Can you work these out from the model? Positions are in its coordinate system, mm. Face numbers are marked on the shaded views. A direction names the side the tool comes from. Give positions to 0.01 mm unless a question says otherwise; leave off trailing zeros. Order: outer loops, then holes, each group sorted by start corner. A loop starts at its lowest first (then second) coordinate and runs counter-clockwise, first axis right, second up. Notation, with made-up numbers: M 31,43 L 69,43 A31 cw 69,78 Z; hole C 64,37.25 d11. An arc over 180 degrees is marked long. Write each question's results on one line, items separated by ' | '.
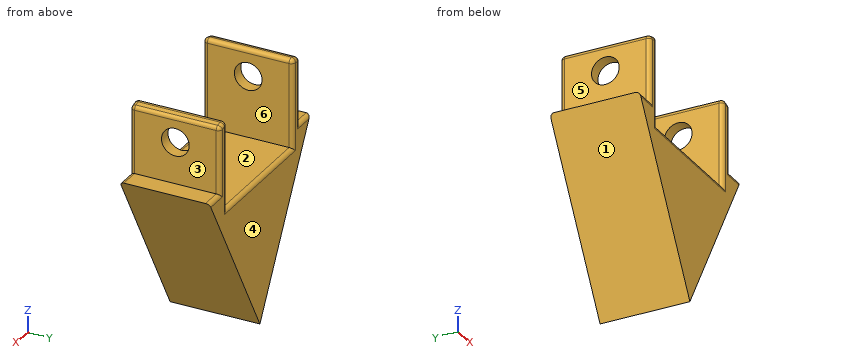
from build123d import *

# Parameters (mm, degrees)
BOSS_EXTRUDE1_DEPTH = 28
CUT_EXTRUDE1_DEPTH  = 90.677477663
SKETCH5_R           = 6.35
CUT_EXTRUDE2_DEPTH  = 4.572
SKETCH8_R           = 6.35
SKETCH8_R_2         = 4.318
BOSS_EXTRUDE4_DEPTH = 6.858
CUT_EXTRUDE6_START  = -2.54
SKETCH13_W          = 36.221601717
SKETCH13_H          = 27.797973411
CUT_EXTRUDE6_DEPTH  = 91.021953984
FILLET3_R           = 1.27


with BuildPart() as part:
    # Sketch2 → Boss-Extrude1 (new body)
    with BuildSketch(Plane(origin=(0, 0, 0), x_dir=(1, 0, 0), z_dir=(0, 1, 0))):
        with BuildLine():
            Line((-38.1, -65.991135768), (0, 0))
            Line((0, 0), (0, -76.2))
            ThreePointArc((0, -76.2), (-19.722011237, -73.603547963), (-38.1, -65.991135768))
        make_face()
    boss_extrude1 = extrude(amount=BOSS_EXTRUDE1_DEPTH)

    # Sketch4 → Cut-Extrude1 (cut, symmetric)
    with BuildSketch(Plane(origin=(0, 28, 0), x_dir=(1, 0, 0), z_dir=(0, 1, 0))):
        Polygon((-19.722011237, -73.603547963), (-19.722011237, -45.603553163), (19.722011237, -45.603553163), (19.722011237, -73.603547963), (19.722011237, -89.083413221), (-19.722011237, -89.083413221), align=None)
    cut_extrude1 = extrude(amount=CUT_EXTRUDE1_DEPTH, both=True, mode=Mode.SUBTRACT)

    # Sketch5 → Cut-Extrude2 (cut)
    with BuildSketch(Plane(origin=(-19.722011237, 0, 0), x_dir=(0, 0, -1), z_dir=(1, 0, 0))):
        with Locations((-64.683550563, 14)):
            Circle(SKETCH5_R)
    cut_extrude2 = extrude(amount=-CUT_EXTRUDE2_DEPTH, mode=Mode.SUBTRACT)

    # Sketch8 → Boss-Extrude4 (add)
    with BuildSketch(Plane(origin=(-19.722011237, 0, 0), x_dir=(0, 0, -1), z_dir=(1, 0, 0))):
        with Locations((-64.683550563, 14)):
            Circle(SKETCH8_R)
        with Locations((-64.683550563, 14)):
            Circle(SKETCH8_R_2, mode=Mode.SUBTRACT)
    boss_extrude4 = extrude(amount=-BOSS_EXTRUDE4_DEPTH)

    # Sketch13 → Cut-Extrude6 (cut)
    with BuildSketch(Plane(origin=(0, 0, 0), x_dir=(1, 0, 0), z_dir=(0, 1, 0)).offset(CUT_EXTRUDE6_START)):
        with Locations((-41.642812096, -65.599005435)):
            Rectangle(SKETCH13_W, SKETCH13_H)
    cut_extrude6 = extrude(amount=CUT_EXTRUDE6_DEPTH, mode=Mode.SUBTRACT)

    # Mirror1: Boss-Extrude1, Cut-Extrude1, Cut-Extrude2, Boss-Extrude4, Cut-Extrude6 across plane
    add(boss_extrude1.mirror(Plane(origin=(0, 28, 0), x_dir=(0, 0, 1), z_dir=(-1, 0, 0))))
    add(cut_extrude1.mirror(Plane(origin=(0, 28, 0), x_dir=(0, 0, 1), z_dir=(-1, 0, 0))), mode=Mode.SUBTRACT)
    add(cut_extrude2.mirror(Plane(origin=(0, 28, 0), x_dir=(0, 0, 1), z_dir=(-1, 0, 0))), mode=Mode.SUBTRACT)
    add(boss_extrude4.mirror(Plane(origin=(0, 28, 0), x_dir=(0, 0, 1), z_dir=(-1, 0, 0))))
    add(cut_extrude6.mirror(Plane(origin=(0, 28, 0), x_dir=(0, 0, 1), z_dir=(-1, 0, 0))), mode=Mode.SUBTRACT)

    # Fillet3
    fillet3_edges = [part.edges().sort_by_distance(p)[0] for p in [
        (21.634365977, 28, 73.064315564),
        (21.634365977, 0, 73.064315564),
        (26.690515484, 0, 51.700018729),
        (0, 0, 45.603553163),
        (23.532011237, 14, 72.475405809),
        (23.532011237, 0, 62.087712269),
        (23.532011237, 28, 62.087712269),
        (26.690515484, 28, 51.700018729),
        (-19.722011237, 0, 59.603550563),
        (-19.722011237, 14, 73.603547963),
        (-19.722011237, 28, 59.603550563),
        (0, 28, 45.603553163),
        (-21.634365977, 0, 73.064315564),
        (-26.690515484, 0, 51.700018729),
        (-21.634365977, 28, 73.064315564),
        (-26.690515484, 28, 51.700018729),
        (-23.532011237, 28, 62.087712269),
        (-23.532011237, 0, 62.087712269),
        (-23.532011237, 14, 72.475405809),
        (19.722011237, 14, 73.603547963),
        (19.722011237, 28, 59.603550563),
        (19.722011237, 0, 59.603550563),
    ]]
    fillet(fillet3_edges, radius=FILLET3_R)


solid = part.part
(1) Imagine slicing it at C-C, the plane y = 24. Write out the boundary of the cut face in (x, z), plus the area to 3 significant figures.
Data:
outline: M -29.85,51.7 L 0,0 L 29.85,51.7 L 23.53,51.7 L 23.53,71.55 A1.27 ccw 22.64,72.76 A76.2 ccw 21.35,73.15 A1.27 ccw 19.72,71.93 L 19.72,45.6 L -19.72,45.6 L -19.72,71.93 A1.27 ccw -21.35,73.15 A76.2 ccw -22.64,72.76 A1.27 ccw -23.53,71.55 L -23.53,51.7 Z | area: 1,460 mm2
(2) Will these pins go through, and if not, where does the flat tip stop? P1, Ø16, axis at y = 10.5, z = 61.5, coming from the -X side; P2, Ø10, axis at x = 4.5, y = 22, coming from the -Z side; P3, Ø2, axis at x = 3, y = 12, coming from the +Z side; P4, Ø5, axis at x = -27.5, y = 10, coming from the +Z side.
Data:
P1: stops at x = -23.53 | P2: stops at z = 0 | P3: stops at z = 45.6 | P4: stops at z = 51.7
(3) We'd pull the mould along X, two halves only. Please class the marked faces 1, 2 and 3: +X half, -X half, draft (parallel to the pull), parting line (faces both ways), or undercut.
Data:
face 1: -X half | face 2: undercut | face 3: +X half
(4) Imagine slicing it at A-A, the plane y = 14. Write out the boundary of the cut face in (x, z), plus the area to 3 significant figures.
Data:
outline: M -29.85,51.7 L 0,0 L 29.85,51.7 L 23.53,51.7 L 23.53,60.37 L 19.72,60.37 L 19.72,45.6 L -19.72,45.6 L -19.72,60.37 L -23.53,60.37 L -23.53,51.7 Z; M -23.53,69 L -19.72,69 L -19.72,71.93 A1.27 ccw -21.35,73.15 A76.2 ccw -22.64,72.76 A1.27 ccw -23.53,71.55 Z; M 19.72,69 L 23.53,69 L 23.53,71.55 A1.27 ccw 22.64,72.76 A76.2 ccw 21.35,73.15 A1.27 ccw 19.72,71.93 Z | area: 1,400 mm2
(5) I need wall thicknesses on L1, parallel to X at y = 20, z = 60; L2, parallel to X at y = 11.5, z = 19; L3, parallel to X at y = 24.5, z = 32. Which ranges of each line are inside material? Lowest first, please. Write a range as from..to.
Data:
L1: x = -23.53..-19.72, 19.72..23.53 | L2: x = -10.97..10.97 | L3: x = -18.48..18.48
(6) Imagine slicing it at D-D, the plane x = -1. Write out the boundary of the cut face in (y, z), plus the area to 3 significant figures.
Data:
outline: M 0,1.73 L 28,1.73 L 28,44.33 A1.27 ccw 26.73,45.6 L 1.27,45.6 A1.27 ccw 0,44.33 Z | area: 1,230 mm2
(7) Imagine slicing it at B-B, the plane z = 58.5. Write out the boundary of the cut face in (x, y), plus the area to 3 significant figures.
Data:
outline: M -23.53,1.27 A1.27 ccw -22.26,0 L -20.99,0 A1.27 ccw -19.72,1.27 L -19.72,26.73 A1.27 ccw -20.99,28 L -22.26,28 A1.27 ccw -23.53,26.73 Z; M 19.72,1.27 A1.27 ccw 20.99,0 L 22.26,0 A1.27 ccw 23.53,1.27 L 23.53,26.73 A1.27 ccw 22.26,28 L 20.99,28 A1.27 ccw 19.72,26.73 Z | area: 211 mm2
(8) For the marked faces 4, 5 and 6, which set-ups out of +Z, -Z, +X, -X, +Y, -Y let a thin tool reach every point of the face, with its end or its side?
Data:
face 4: +Z, -Z, +X, -X, +Y | face 5: +Z, -X, +Y, -Y | face 6: +Z, +Y, -Y
